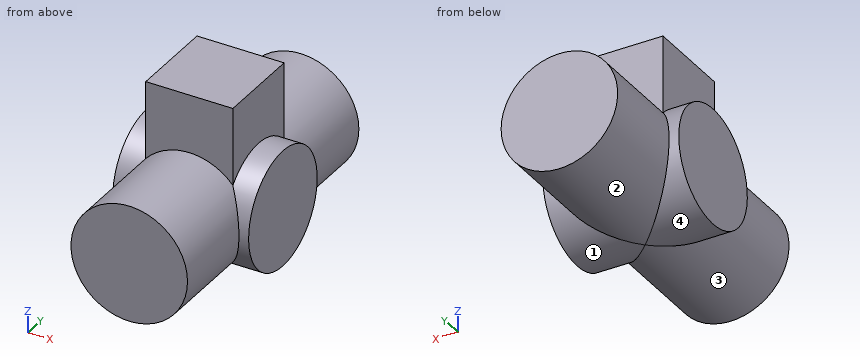
from build123d import *

# Parameters (mm, degrees)
SKETCH1_R           = 30
BOSS_EXTRUDE1_DEPTH = 150
SKETCH3_R           = 30
BOSS_EXTRUDE2_DEPTH = 35
BOSS_EXTRUDE3_DEPTH = 60


with BuildPart() as part:
    # Sketch1 → Boss-Extrude1 (new body)
    with BuildSketch(Plane(origin=(0, 0, 0), x_dir=(1, 0, 0), z_dir=(0, 1, 0))):
        Circle(SKETCH1_R)
    extrude(amount=BOSS_EXTRUDE1_DEPTH)

    # Sketch3 → Boss-Extrude2 (add, symmetric)
    with BuildSketch(Plane(origin=(0, 0, 0), x_dir=(0, 0, -1), z_dir=(1, 0, 0))):
        with Locations((0, 75)):
            Circle(SKETCH3_R)
    extrude(amount=BOSS_EXTRUDE2_DEPTH, both=True)

    # Sketch4 → Boss-Extrude3 (add)
    with BuildSketch(Plane.XY):
        Polygon((0, 97.430213505), (22.430213505, 97.430213505), (22.430213505, 52.569786495), (-22.430213505, 52.569786495), (-22.430213505, 97.430213505), align=None)
    extrude(amount=BOSS_EXTRUDE3_DEPTH)


solid = part.part
Build history of the part. All positions in model axes, mm. Face numbers are marked on the shaded views. A direction names the side the tool comes from. Coordinates: 2 decimals unless noted, no trailing zeros. Write each loop counter-clockwise with the first axis right and the second up, starting at its lowest first coordinate (ties: lowest second). Pieces come first, ordered by that corner, then holes.
(1) Drill centre lines: line 1 (X direction, y = 80, z = 31); line 2 (Y direction, x = 5, z = 32.5); line 3 (Z direction, x = 24.5, y = 74.5). Where is each one in solid material? Low to high.
(2) Cut at C-C on y = 87. List the corners of the cut face in (x, z), and give its area (3 significant figures).
(3) Cut at D-D on z = 24.5. List the corners of the cut face in (x, y), and give its area (3 significant figures).
(4) Cut at A-A on z = 0. List the corners of the cut face in (x, y).
(5) Pin check, flat tips, straight feed: pin 1 Ø2 at (x, y) = (27.5, 70) entering from -Z; pin 2 Ø2 at (x, y) = (-12, 121) entering from -Z; pin 3 Ø3 at (x, y) = (14.5, 77) entering from -Z. Stop position of each tip, or through.
(6) 3-axis set-ups, long thin cutter, end or side, ignore diameter. For the marked faces 1, 2, 3 and 4: which of +Z, -Z, +X, -X, +Y, -Y reach the whole face in a straight line?
(7) Cut at B-B on x = -13.5. List the corners of the cut face in (y, z), and give its area (3 significant figures).
Working result:
1. line 1: x = -22.43 to 22.43
1. line 2: y = 52.57 to 97.43
1. line 3: z = -30 to 30
2. outline: (-35, -27.5) - (-12, -27.5) arc R30 ccw to (12, -27.5) - (35, -27.5) - (35, 27.5) - (22.43, 27.5) - (22.43, 60) - (-22.43, 60) - (-22.43, 27.5) - (-35, 27.5) - close
2. area: 5,350 mm2
3. outline: (-35, 57.69) - (-22.43, 57.69) - (-22.43, 52.57) - (-17.31, 52.57) - (-17.31, 0) - (17.31, 0) - (17.31, 52.57) - (22.43, 52.57) - (22.43, 57.69) - (35, 57.69) - (35, 92.31) - (22.43, 92.31) - (22.43, 97.43) - (17.31, 97.43) - (17.31, 150) - (-17.31, 150) - (-17.31, 97.43) - (-22.43, 97.43) - (-22.43, 92.31) - (-35, 92.31) - close
3. area: 6,520 mm2
4. outline: (-35, 45) - (-30, 45) - (-30, 0) - (30, 0) - (30, 45) - (35, 45) - (35, 105) - (30, 105) - (30, 150) - (-30, 150) - (-30, 105) - (-35, 105) - close
5. pin 1: stops at z = -29.73
5. pin 2: stops at z = -27.91
5. pin 3: stops at z = -30
6. face 1: +X
6. face 2: +Y
6. face 3: -Y
6. face 4: -X
7. outline: (0, -26.79) - (61.5, -26.79) arc R30 ccw to (88.5, -26.79) - (150, -26.79) - (150, 26.79) - (97.43, 26.79) - (97.43, 60) - (52.57, 60) - (52.57, 26.79) - (0, 26.79) - close
7. area: 9,590 mm2
